Part model, mm, in its own coordinate system. A direction names the side the tool comes from. Coordinates: 2 decimals unless noted, no trailing zeros. Loops run counter-clockwise (first coordinate to the right, second up) from the corner with the lowest first, then second, coordinate; pieces in that order, holes last. Notation, with made-up numbers: (-9.5, -11.75) - (17.5, -11.75) arc R35 cw to (17.5, 21.25) - close; hole circle Ø6 at (-36.5, 33.5). An arc over 180 degrees is marked (long way). Use a Markdown table: item, result. Add a question column.
1) Pull direction Z, two halves, no side cores. Call faces 5 (the face through (3, 23, 0)), 6 (the face through (3.4, 0.5, 20.8)), 7 (the face through (-6.921, 21.344, 7.888)): +Z half, -Z half, draft (parallel to the pull), parting line (faces both ways), or undercut.
2) Probe probe 1 along Z at (x, y) = (5, 0.8); probe 2 along X at (y, z) = (0.8, 22); probe 3 along Z at (x, y) = (-3, 28.5). List the from-to ranges inside material, lowest first. Write a range as [from, to].
3) Drop flat-ended pins along their axis: P1, Ø1, axis at x = 2, z = 22, coming from the +Y side; P2, Ø3.5, axis at y = 1, z = 5.5, coming from the -X side; P3, Ø3, axis at x = 5, z = 22, coming from the +Y side; P4, Ø10, axis at y = 8.5, z = 13, coming from the +X side. Give the stop position or say it passes through.
4) Tool access for faces 1 (the face through (6, 3, 8)), 2 (the face through (0, 1, 8)), 3 (the face through (3, 23, 16)), 4 (the face through (3.83, 18.45, 7.89)): list every direction of +Z, -Z, +X, -X, +Y, -Y with a clear straight run to the whole face (end or side of a thin tool).
5) Band-saw the part on A-A (z = 22). Give the cut face in (x, y), plus the area to 3 significant figures.
6) Band-saw the part on B-B (z = 11.5). Give the cut face in (x, y).
7) Band-saw the part on C-C (x = -0.5). Give the cut face in (y, z), plus the area to 3 significant figures.
8) Band-saw the part on D-D (y = 7.5). Give the cut face in (x, z).
from build123d import *

# Parameters (mm, degrees)
F1_DEPTH       = 16
F2_W           = 9.5
F2_H           = 3
F3_DEPTH       = 11
F6_D           = 4
F6_CSINK_D     = 8
F6_CSINK_ANGLE = 90
F8_R           = 2
F9_R           = 3
F10_R          = 2


with BuildPart() as f1:
    # F0 (on Top) → F1 (new body)
    with BuildSketch(Plane.XY):
        with BuildLine():
            ThreePointArc((2, 3), (3.5524079534, 17.0474266553), (7.2489157042, 30.688394236))
            ThreePointArc((7.2489157042, 30.688394236), (6.4110728807, 33.0634017317), (3.9140154247, 32.735765863))
            ThreePointArc((3.9140154247, 32.735765863), (-0.2014778431, 29.7072757815), (-5.1119606936, 28.2944080641))
            ThreePointArc((-5.1119606936, 28.2944080641), (-6.1052113837, 27.8706276086), (-6.6852554951, 26.9597567962))
            Line((-6.6852554951, 26.9597567962), (-7.7398444423, 23.101280134))
            ThreePointArc((-7.7398444423, 23.101280134), (-6.8937110874, 21.3313839825), (-5.019957521, 21.9123500865))
            Line((-5.019957521, 21.9123500865), (-2.5832541287, 25.8215889335))
            Line((-2.5832541287, 25.8215889335), (0, 26.3843059314))
            ThreePointArc((0, 26.3843059314), (1.8642632491, 25.8195517282), (2.3638801074, 23.9367857399))
            ThreePointArc((2.3638801074, 23.9367857399), (0.4646962608, 13.5493737022), (0, 3))
            Line((0, 3), (0, 0))
            Line((0, 0), (9.5, 0))
            Line((9.5, 0), (9.5, 3))
            Line((9.5, 3), (2, 3))
        make_face()
    extrude(amount=F1_DEPTH)

    # F2 (on face) → F3 (join)
    with BuildSketch(Plane.XY.offset(16)):
        with Locations((4.75, 1.5)):
            Rectangle(F2_W, F2_H)
    extrude(amount=F3_DEPTH)

    # F6 (through all)
    with Locations(Plane(origin=(0, 3, 0), x_dir=(-1, 0, 0), z_dir=(0, 1, 0))):
        with Locations((-5, 22)):
            CounterSinkHole(F6_D / 2, F6_CSINK_D / 2, counter_sink_angle=F6_CSINK_ANGLE)

    # F7: F1 across plane


with BuildPart() as f1_1:
    add(f1.part)
    add(f1.part.mirror(Plane.XY.offset(8)))

    # F8
    f8_edges = [f1_1.edges().sort_by_distance(p)[0] for p in [
        (0, 1.5, 27),
        (0, 1.5, -11),
    ]]
    fillet(f8_edges, radius=F8_R)

    # F9
    f9_edges = [f1_1.edges().sort_by_distance(p)[0] for p in [
        (2, 3, 8),
    ]]
    fillet(f9_edges, radius=F9_R)

    # F10
    f10_edges = [f1_1.edges().sort_by_distance(p)[0] for p in [
        (-2.583254, 25.821589, 8),
    ]]
    fillet(f10_edges, radius=F10_R)


solid = f1_1.part
Answer block:
| question | item | result |
|---|---|---|
| 1 | face 5 | -Z half |
| 1 | face 6 | undercut |
| 1 | face 7 | draft |
| 2 | probe 1 | [-11, -8], [-4, 20], [24, 27] |
| 2 | probe 2 | [0, 3], [7, 9.5] |
| 2 | probe 3 | [0, 16] |
| 3 | P1 | y = 2.5 |
| 3 | P2 | x = 0 |
| 3 | P3 | through |
| 3 | P4 | x = 3.5 |
| 4 | face 1 | +X |
| 4 | face 2 | +Z, -Z, -X, -Y |
| 4 | face 3 | +Z, +X, -X, +Y |
| 4 | face 4 | +Z, -Z, +X |
| 5 | outline | (0, 0) - (3, 0) - (3, 1) - (1, 3) - (0, 3) - close; (7, 0) - (9.5, 0) - (9.5, 3) - (9, 3) - (7, 1) - close |
| 5 | area | 12.5 mm2 |
| 6 | outline | (-7.74, 23.1) arc R1.5 ccw to (-5.02, 21.91) - (-3.03, 25.11) arc R2 cw to (-1.76, 26) - (0, 26.38) arc R2 cw to (2.36, 23.94) arc R77.24 ccw to (0, 3) - (0, 0) - (9.5, 0) - (9.5, 3) - (5.15, 3) arc R3 cw to (2.16, 6.2) arc R91.53 cw to (7.25, 30.69) arc R2 ccw to (3.91, 32.74) arc R14.5 cw to (-5.11, 28.29) arc R1.83 ccw to (-6.69, 26.96) - close |
| 7 | outline | (26.28, 0) - (29.56, 0) - (29.56, 16) - (26.28, 16) - close |
| 7 | area | 52.6 mm2 |
| 8 | outline | (0.02, 0) - (2.26, 0) - (2.26, 16) - (0.02, 16) - close |
